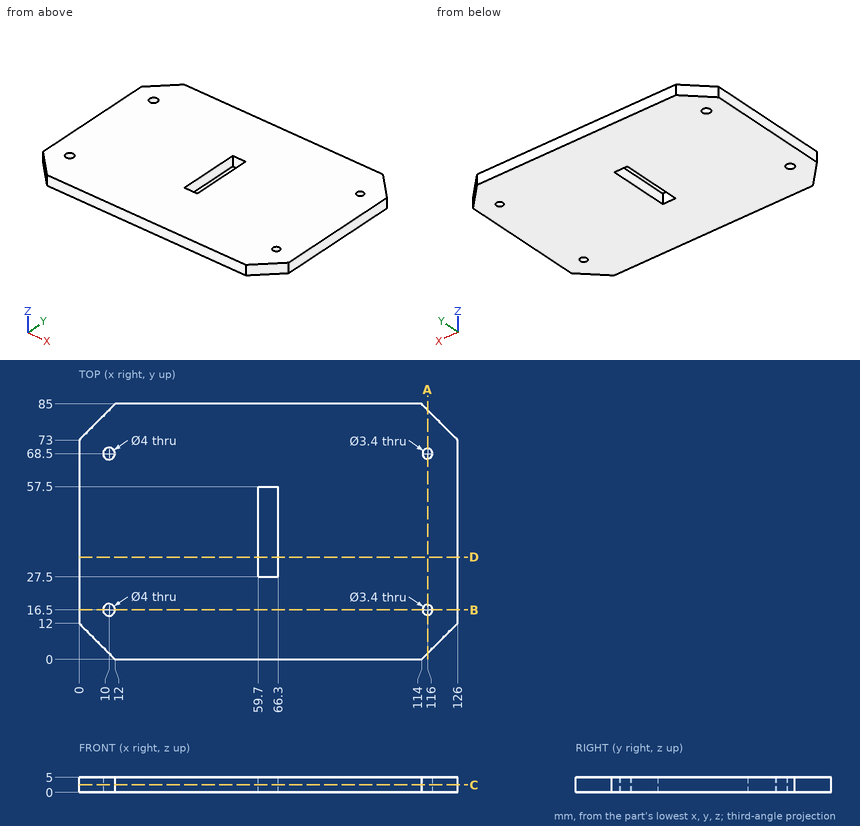
Can you work these out from the drawing? Everything is in mm from the part's minimum corner. Round coordinates to 2 decimals unless told otherwise and drop trailing zeros. Loops run counter-clockwise (first coordinate to the right, second up) from the corner with the lowest first, then second, coordinate; pieces in that order, holes last. Notation, with made-up numbers: M 8.5,-20.5 L 50.5,-20.5 A25 ccw 50.5,6.5 Z; hole C 24,-27.75 d11. An arc over 180 degrees is marked long. Answer in a Markdown table with one row per item.
1. If we section it at B-B, the plane y = 16.5: Please give me the cut outline in (x, z).
Established:
| item | result |
|---|---|
| outline | M 0,0 L 8,0 L 8,5 L 0,5 Z; M 12,0 L 114.3,0 L 114.3,5 L 12,5 Z; M 117.7,0 L 126,0 L 126,5 L 117.7,5 Z |
2. I'm going to push flat-ended pins straight in: pin 1 Ø5 at (x, y) = (10, 68.5) entering from -Z; pin 2 Ø2 at (x, y) = (62.5, 39) entering from -Z. Where does each tip first touch, or does it pass through?
Established:
| item | result |
|---|---|
| pin 1 | z = 0 |
| pin 2 | through |
3. Please list where these lines run through material, in increasing order: line 1 (X direction, y = 68.5, z = 1.15); line 2 (X direction, y = 54.5, z = 4.45); line 3 (Y direction, x = 65, z = 3.8). Write a range as from..to.
Established:
| item | result |
|---|---|
| line 1 | 0..8, 12..114.3, 117.7..126 |
| line 2 | 0..59.7, 66.3..126 |
| line 3 | 0..27.5, 57.5..85 |
4. If we section it at D-D, the plane y = 34: Please give me the cut outline in (x, z), plus the area to 3 significant figures.
Established:
| item | result |
|---|---|
| outline | M 0,0 L 59.7,0 L 59.7,5 L 0,5 Z; M 66.3,0 L 126,0 L 126,5 L 66.3,5 Z |
| area | 597 mm² |
5. If we section it at C-C, the plane z = 2.55: Please give me the cut outline in (x, y), plus the area to 3 significant figures.
Established:
| item | result |
|---|---|
| outline | M 0,12 L 12,0 L 114,0 L 126,12 L 126,73 L 114,85 L 12,85 L 0,73 Z; hole C 10,16.5 d4; hole C 10,68.5 d4; hole M 59.7,27.5 L 66.3,27.5 L 66.3,57.5 L 59.7,57.5 Z; hole C 116,16.5 d3.4; hole C 116,68.5 d3.4 |
| area | 10,200 mm² |
6. If we section it at A-A, the plane x = 116: Please give me the cut outline in (y, z).
Established:
| item | result |
|---|---|
| outline | M 2,0 L 14.8,0 L 14.8,5 L 2,5 Z; M 18.2,0 L 66.8,0 L 66.8,5 L 18.2,5 Z; M 70.2,0 L 83,0 L 83,5 L 70.2,5 Z |
